Job drawing, mm, ordinate dimensions from the low corner. One solid piece. A direction names the side the tool comes from. Round coordinates to 2 decimals unless told otherwise and drop trailing zeros. Order: outer loops, then holes, each group sorted by start corner. A loop starts at its lowest first (then second) coordinate and runs counter-clockwise, first axis right, second up. Notation, with made-up numbers: M 81.5,68 L 106.5,68 A14 cw 106.5,83 Z; hole C 24,61 d10. An arc over 180 degrees is marked long. Answer as a JSON object with one key per item and string values. Group by question number.
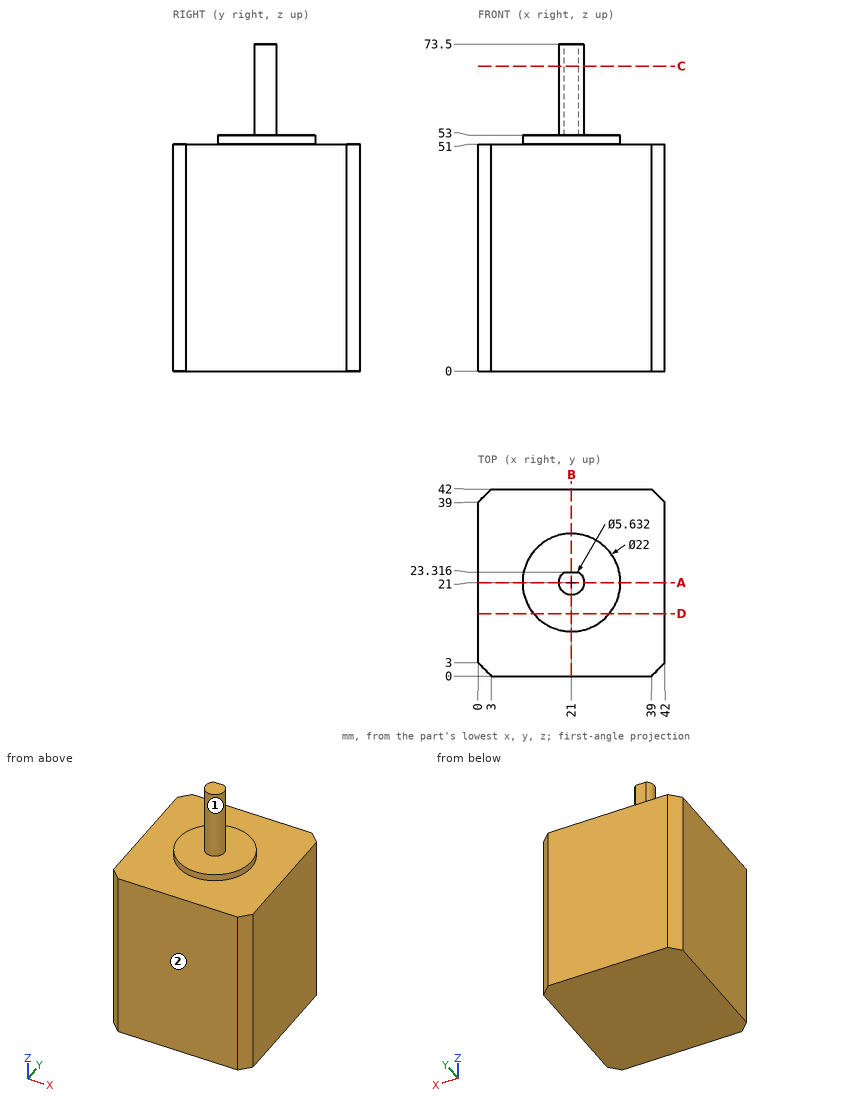
Item 1: Flat gauge pins, fed straight in: pin 1 Ø1.6 at (x, z) = (21.5, 60.5) entering from +Y; pin 2 Ø5 at (x, y) = (18, 35.5) entering from +Z; pin 3 Ø2 at (x, y) = (23, 15.5) entering from +Z. Where does each tip first touch, or does it go through?
Item 2: Cut at B-B, the plane x = 21. Give the cut face in (y, z).
Item 3: 3-axis set-ups, long thin cutter, end or side, ignore diameter. For the marked faces 1 and 2: which of +Z, -Z, +X, -X, +Y, -Y reach the whole face in a straight line?
Item 4: Cut at D-D, the plane y = 14. Give the cut face in (x, z) (1 decimal).
Item 5: Cut at C-C, the plane z = 68.5. Give the cut face in (x, y), and give its area (3 significant figures).
Item 6: Cut at A-A, the plane y = 21. Give the cut face in (x, z).
Item 7: Drill centre lines: line 1 (Z direction, x = 30, y = 14); line 2 (Z direction, x = 29, y = 24); line 3 (Y direction, x = 18.5, z = 67.5) (1 decimal). Where is each one in solid material? Low to high. Write a range as [from, to].
Response values:
{
 "1": {"pin 1": "y = 23.32", "pin 2": "z = 51", "pin 3": "z = 53"},
 "2": {"outline": "M 0,0 L 42,0 L 42,51 L 32,51 L 32,53 L 23.32,53 L 23.32,73.5 L 18.18,73.5 L 18.18,53 L 10,53 L 10,51 L 0,51 Z"},
 "3": {"face 1": "+Z", "face 2": "+Z, -Z, +X, -X, -Y"},
 "4": {"outline": "M 0,0 L 42,0 L 42,51 L 29.5,51 L 29.5,53 L 12.5,53 L 12.5,51 L 0,51 Z"},
 "5": {"outline": "M 19.4,23.32 A2.82 ccw long 22.6,23.32 Z", "area": "23.8 mm^2"},
 "6": {"outline": "M 0,0 L 42,0 L 42,51 L 32,51 L 32,53 L 23.82,53 L 23.82,73.5 L 18.18,73.5 L 18.18,53 L 10,53 L 10,51 L 0,51 Z"},
 "7": {"line 1": "[0, 51]", "line 2": "[0, 53]", "line 3": "[19.7, 22.3]"}
}
